Check sheet for the modelled part. Datum: model origin and axes. Units: mm. A direction names the side the tool comes from. Give positions to 0.01 mm unless a question says otherwise; leave off trailing zeros. Write each loop counter-clockwise with the first axis right and the second up, starting at its lowest first coordinate (ties: lowest second). Pieces come first, ordered by that corner, then holes. Notation, with made-up numbers: (55, 13) -> (95, 13) arc R35 cw to (95, 45) -> close; hole circle Ø9 at (39, 45.5). An arc over 180 degrees is marked (long way). Answer as a JSON object with one key per item and string values.
Autodesk Inventor part; units mm, degrees
ref_plane "YZ Plane" through (0, 0, 0) normal (1, 0, 0) x (0, 1, 0)
ref_plane "XZ Plane" through (0, 0, 0) normal (0, 1, 0) x (-1, 0, 0)
ref_plane "XY Plane" through (0, 0, 0) normal (0, 0, 1) x (1, 0, 0)
sketch "Sketch1" plane through (0, 0, 0) normal (0, 0, 1) x (1, 0, 0)
  circle A0 centre (0, 0) radius 7.9375
  circle A1 centre (0, 0) radius 13.6922
  dimension "d0" = 15.875
  dimension "d1" = 27.3844
extrude "Extrusion1" add sketch "Sketch1" along normal blind 43.6562
ref_plane "Work Plane1" through (0, 0, 21.8281) normal (0, 0, 1) x (1, 0, 0)
sketch "Sketch3" plane through (0, 0, 21.8281) normal (0, 0, 1) x (1, 0, 0)
  circle A0 centre (0, 0) radius 7.9375
extrude "Extrusion2" add sketch "Sketch3" along normal mid plane 12.7
sketch "Sketch5" plane through (0, 0, 0) normal (0, 0, -1) x (-1, 0, 0)
  circle A0 centre (0, 0) radius 3.175
  circle A1 centre (0, 0) radius 13.6922
  circle A2 centre (0, 0) radius 7.9375
  dimension "d6" = 6.35
extrude "Extrusion3" add sketch "Sketch5" against normal up to surface (15.4781 mm away) contours A2
properties part number "Machinable Bore Flexible Shaft Coupling"
1. Sectioned sample at D-D, the plane z = 26. Enter the section's corners in (x, y).
Determined:
{"outline": "circle Ø27.38 at (0, 0)"}
2. Sectioned sample at A-A, the plane y = 0. Enter the section's corners in (x, z) (1 decimal).
Determined:
{"outline": "(-13.7, 0) -> (-3.2, 0) -> (-3.2, 15.5) -> (3.2, 15.5) -> (3.2, 0) -> (13.7, 0) -> (13.7, 43.7) -> (7.9, 43.7) -> (7.9, 28.2) -> (-7.9, 28.2) -> (-7.9, 43.7) -> (-13.7, 43.7) -> close"}
3. Sectioned sample at C-C, the plane z = 15. Enter the section's corners in (x, y) (3 decimals).
Determined:
{"outline": "circle Ø27.384 at (0, 0); hole circle Ø6.35 at (0, 0)"}
4. Scan lines: L1, parallel to Y at x = 0, z = 32; L2, parallel to Y at x = 0, z = 6 (3 decimals); L3, parallel to Z at x = -3, y = 6.25. Record each from-to range of solid material in increasing order. Write a range as [from, to].
Determined:
{"L1": "[-13.69, -7.94], [7.94, 13.69]", "L2": "[-13.692, -3.175], [3.175, 13.692]", "L3": "[0, 28.18]"}
5. Go/stop test with flat-tipped pins: P1, Ø1.5, axis at y = -7, z = 31.5, coming from the -X side; P2, Ø6, axis at x = 8, z = 38.5, coming from the -Y side; P3, Ø8.5, axis at x = 0, y = 0, coming from the +Z side; P4, Ø12, axis at x = -2.5, y = -1, coming from the -Z side. Record where each tip stops, or that it passes through.
Determined:
{"P1": "x = -12.18", "P2": "y = -12.75", "P3": "z = 28.18", "P4": "z = 0"}
6. Mould release check, pull along Y, two halves, no side actions. Record for faces 4 (the face through (-2.968, 13.367, 21.523)), 5 (the face through (-3, -3, 0)), 6 (the face through (-1.72, 7.75, 35.81)): released by +Y, released by -Y, zero draft, split by the parting line, or undercut.
Determined:
{"face 4": "split by the parting line", "face 5": "zero draft", "face 6": "undercut"}
7. Access from +Z, -Z, +X, -X, +Y, -Y to the whole of each face (thin tool, end or side, straight path). Record for faces 1 (the face through (6, -6, 43.656)), 2 (the face through (0, 0, 15.478)), 3 (the face through (0, 0, 28.178)).
Determined:
{"face 1": "+Z, +X, -X, +Y, -Y", "face 2": "-Z", "face 3": "+Z"}
